Can you work these out from the model? Positions are in its coordinate system, mm. Give positions to 0.01 mm unless a question says otherwise; leave off trailing zeros. Loops run counter-clockwise (first coordinate to the right, second up) from the corner with the lowest first, then second, coordinate; pieces in that order, holes last. Notation, with made-up numbers: (21, 71) - (25, 71) arc R19 ccw to (25, 81) - close; hole circle Ø4 at (-35, 48.5). An arc over 180 degrees is marked (long way). Answer as a JSON object with one key per item and string values.
```python
from build123d import *

# Parameters (mm, degrees)
Y_KSEKLIK_EKSTR_ZYON1_DEPTH = 2
RADYUS1_R                   = 10
RADYUS2_R                   = 3
IZIM2_W                     = 2.1
IZIM2_H                     = 28
KES_EKSTR_ZYON1_DEPTH       = 10
KES_EKSTR_ZYON2_DEPTH       = 10
KES_EKSTR_ZYON3_DEPTH       = 10
IZIM5_R                     = 6.1
KES_EKSTR_ZYON4_DEPTH       = 10
IZIM6_R                     = 1.6
KES_EKSTR_ZYON5_DEPTH       = 10


with BuildPart() as part:
    # Çizim1 → Yükseklik-Ekstrüzyon1 (new body)
    with BuildSketch(Plane.XY):
        Polygon((78.397764574, 53), (78.397764574, 58), (-79.202235426, 58), (-79.202235426, 53), (-79.202235426, 4.7), (-99.202235426, 4.7), (-99.202235426, -129.7), (-79.202235426, -129.7), (-79.202235426, -178), (-79.202235426, -183), (78.397764574, -183), (78.397764574, -178), (78.397764574, -129.7), (98.397764574, -129.7), (98.397764574, 4.7), (78.397764574, 4.7), align=None)
    extrude(amount=Y_KSEKLIK_EKSTR_ZYON1_DEPTH)

    # Radyus1
    radyus1_edges = [part.edges().sort_by_distance(p)[0] for p in [
        (-79.202235426, 58, 1),
        (78.397764574, 58, 1),
        (98.397764574, 4.7, 1),
        (98.397764574, -129.7, 1),
        (78.397764574, -183, 1),
        (-79.202235426, -183, 1),
        (-99.202235426, -129.7, 1),
        (-99.202235426, 4.7, 1),
    ]]
    fillet(radyus1_edges, radius=RADYUS1_R)

    # Radyus2
    radyus2_edges = [part.edges().sort_by_distance(p)[0] for p in [
        (78.397764574, 4.7, 1),
        (78.397764574, -129.7, 1),
        (-79.202235426, -129.7, 1),
        (-79.202235426, 4.7, 1),
    ]]
    fillet(radyus2_edges, radius=RADYUS2_R)

    # Çizim2 → Kes-Ekstrüzyon1 (cut)
    with BuildSketch(Plane(origin=(0, 0, 0), x_dir=(-1, 0, 0), z_dir=(0, 0, -1))):
        with Locations((-58.547764574, -159.55)):
            Rectangle(IZIM2_W, IZIM2_H)
        with Locations((59.352235426, -159.55)):
            Rectangle(IZIM2_W, IZIM2_H)
        with Locations((59.352235426, 34.55)):
            Rectangle(IZIM2_W, IZIM2_H)
        with Locations((-58.547764574, 34.55)):
            Rectangle(IZIM2_W, IZIM2_H)
    extrude(amount=-KES_EKSTR_ZYON1_DEPTH, mode=Mode.SUBTRACT)

    # Çizim3 → Kes-Ekstrüzyon2 (cut)
    with BuildSketch(Plane(origin=(0, 0, 0), x_dir=(-1, 0, 0), z_dir=(0, 0, -1))):
        with BuildLine():
            Line((39.202235426, -171), (-38.397764574, -171))
            ThreePointArc((-38.397764574, -171), (-45.468832385, -168.071067812), (-48.397764574, -161))
            Line((-48.397764574, -161), (-48.397764574, -91))
            ThreePointArc((-48.397764574, -91), (-45.468832385, -83.928932188), (-38.397764574, -81))
            Line((-38.397764574, -81), (39.202235426, -81))
            ThreePointArc((39.202235426, -81), (46.273303238, -83.928932188), (49.202235426, -91))
            Line((49.202235426, -91), (49.202235426, -161))
            ThreePointArc((49.202235426, -161), (46.273303238, -168.071067812), (39.202235426, -171))
        make_face()
    extrude(amount=-KES_EKSTR_ZYON2_DEPTH, mode=Mode.SUBTRACT)

    # Çizim4 → Kes-Ekstrüzyon3 (cut)
    with BuildSketch(Plane(origin=(0, 0, 0), x_dir=(-1, 0, 0), z_dir=(0, 0, -1))):
        with BuildLine():
            Line((29.202235426, -71), (-28.397764574, -71))
            ThreePointArc((-28.397764574, -71), (-35.468832385, -68.071067812), (-38.397764574, -61))
            Line((-38.397764574, -61), (-38.397764574, 28))
            ThreePointArc((-38.397764574, 28), (-35.468832385, 35.071067812), (-28.397764574, 38))
            Line((-28.397764574, 38), (29.202235426, 38))
            ThreePointArc((29.202235426, 38), (36.273303238, 35.071067812), (39.202235426, 28))
            Line((39.202235426, 28), (39.202235426, -61))
            ThreePointArc((39.202235426, -61), (36.273303238, -68.071067812), (29.202235426, -71))
        make_face()
    extrude(amount=-KES_EKSTR_ZYON3_DEPTH, mode=Mode.SUBTRACT)

    # Çizim5 → Kes-Ekstrüzyon4 (cut)
    with BuildSketch(Plane(origin=(0, 0, 0), x_dir=(-1, 0, 0), z_dir=(0, 0, -1))):
        with Locations((-63.397764574, -62)):
            Circle(IZIM5_R)
    extrude(amount=-KES_EKSTR_ZYON4_DEPTH, mode=Mode.SUBTRACT)

    # Çizim6 → Kes-Ekstrüzyon5 (cut)
    with BuildSketch(Plane(origin=(0, 0, 0), x_dir=(-1, 0, 0), z_dir=(0, 0, -1))):
        with Locations((49.202235426, -175)):
            Circle(IZIM6_R)
        with Locations((56.202235426, -138)):
            Circle(IZIM6_R)
        with Locations((1.202235426, -76)):
            Circle(IZIM6_R)
        with Locations((1.202235426, -178)):
            Circle(IZIM6_R)
        with Locations((92.202235426, -99.7)):
            Circle(IZIM6_R)
        with Locations((92.202235426, -25.3)):
            Circle(IZIM6_R)
        with Locations((56.202235426, 13)):
            Circle(IZIM6_R)
        with Locations((49.202235426, 50)):
            Circle(IZIM6_R)
        with Locations((-48.397764574, 50)):
            Circle(IZIM6_R)
        with Locations((-55.397764574, 13)):
            Circle(IZIM6_R)
        with Locations((-91.397764574, -25.3)):
            Circle(IZIM6_R)
        with Locations((-91.397764574, -99.7)):
            Circle(IZIM6_R)
        with Locations((-55.397764574, -138)):
            Circle(IZIM6_R)
        with Locations((-48.397764574, -175)):
            Circle(IZIM6_R)
    extrude(amount=-KES_EKSTR_ZYON5_DEPTH, mode=Mode.SUBTRACT)


solid = part.part
```
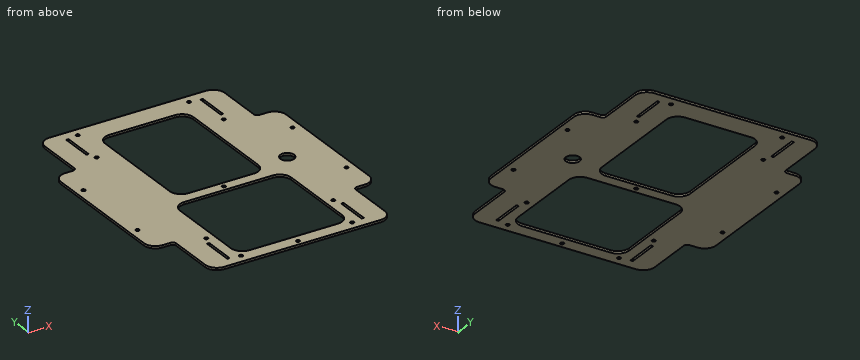
1) I'm going to push flat-ended pins straight in: P1, Ø0.6, axis at x = 86.5, z = 1, coming from the -Y side; P2, Ø1, axis at y = 19.5, z = 1, coming from the +X side. Where does each tip first touch, or does it pass through?
Check sheet entries:
{"P1": "y = -129.7", "P2": "x = 78.4"}
2) Imagine slicing it at B-B on y = -94.5. Write out the boundary of the cut face in (x, z).
Check sheet entries:
{"outline": "(-99.2, 0) - (-49.2, 0) - (-49.2, 2) - (-99.2, 2) - close; (48.4, 0) - (98.4, 0) - (98.4, 2) - (48.4, 2) - close"}
3) Imagine slicing it at A-A on y = 40.5. Write out the boundary of the cut face in (x, z), and give its area (3 significant figures).
Check sheet entries:
{"outline": "(-79.2, 0) - (-60.4, 0) - (-60.4, 2) - (-79.2, 2) - close; (-58.3, 0) - (57.5, 0) - (57.5, 2) - (-58.3, 2) - close; (59.6, 0) - (78.4, 0) - (78.4, 2) - (59.6, 2) - close", "area": "307 mm2"}
4) Imagine slicing it at D-D on y = -125.5. Write out the boundary of the cut face in (x, z).
Check sheet entries:
{"outline": "(-97.35, 0) - (-49.2, 0) - (-49.2, 2) - (-97.35, 2) - close; (48.4, 0) - (96.54, 0) - (96.54, 2) - (48.4, 2) - close"}
5) Imagine slicing it at C-C on z = 1.15. Give the number of separate pieces and of enclosed holes in the cut face, and give its area (3 significant figures).
Check sheet entries:
{"separate pieces": "1", "enclosed holes": "21", "area": "25,700 mm2"}
6) I need wall thicknesses on L1, parallel to Y at x = -18, z = 1.15; L2, parallel to X at y = 47.5, z = 0.75; L3, parallel to X at y = -175, z = 0.5. Which ranges of each line are inside material? Lowest first, please.
Check sheet entries:
{"L1": "-183 to -171, -81 to -71, 38 to 58", "L2": "-79.2 to -60.4, -58.3 to 57.5, 59.6 to 78.4", "L3": "-79 to -50.8, -47.6 to 46.8, 50 to 78.2"}
